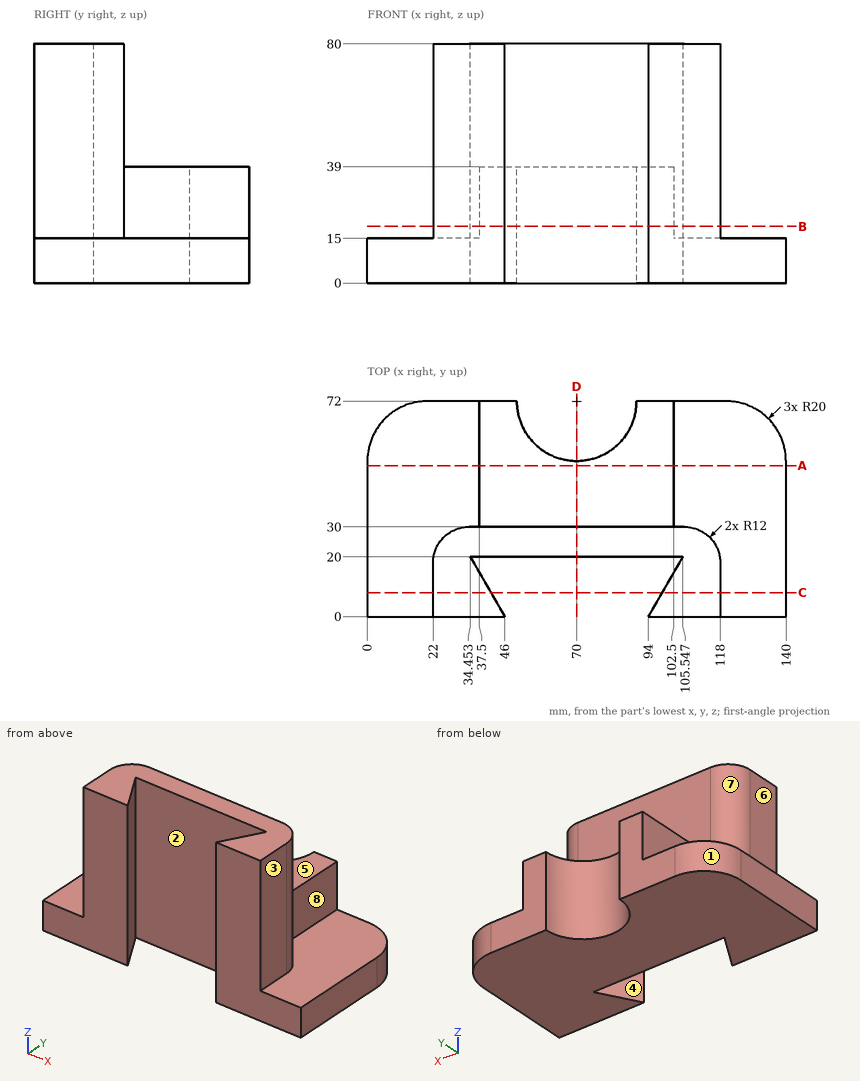
Could you check a few things on this drawing? It's one solid part, dimensions in mm from its lowest x, y, z. A direction names the side the tool comes from. Round coordinates to 2 decimals unless told otherwise and drop trailing zeros. Order: outer loops, then holes, each group sorted by start corner. A loop starts at its lowest first (then second) coordinate and runs counter-clockwise, first axis right, second up. Notation, with made-up numbers: M 42.5,37 L 76.5,37 A29 cw 76.5,76 Z; hole C 61,-5 d2. An arc over 180 degrees is marked long. Return JSON: item names as keys, results as strings. Group by question number.
1. I'm going to push flat-ended pins straight in: pin 1 Ø7 at (y, z) = (56.5, 29.5) entering from +X; pin 2 Ø12 at (x, y) = (59.5, 38) entering from -Z; pin 3 Ø12 at (y, z) = (48, 27) entering from -X; pin 4 Ø5.5 at (y, z) = (5.5, 42.5) entering from +X. Where does each tip first touch, or does it pass through?
2. If we section it at A-A on y = 50.5: List the corners of the cut face in (x, z) for me, then the cut area to 3 significant figures.
3. If we section it at B-B on z = 19: List the corners of the cut face in (x, y) for me.
4. If we mould it in two halves opening along Y, with no side actions, what happens to the marked faces 1, 2 and 3? For each: pulls with the +Y half, pulls with the -Y half, needs draft (parallel to the pull), parting line crosses it, or undercut.
5. Please list where these lines run through material, in increasing order: probe 1 along Y at (x, z) = (84.5, 62); probe 2 along X at (y, z) = (14.5, 11); probe 3 along Z at (x, y) = (72, 36).
6. On a 3-axis mill with a long thin cutter (end or side, diameter ignored), from which of +Z, -Z, +X, -X, +Y, -Y can I reach the whole of each face in a straight line? I mean the marked faces 4, 5, 6, 7 and 8. Say none if no direction works.
7. If we section it at C-C on y = 8: List the corners of the cut face in (x, z) for me.
8. If we section it at D-D on x = 70: List the corners of the cut face in (y, z) for me, then the cut area to 3 significant figures.
Reply:
{
 "1": {"pin 1": "x = 102.5", "pin 2": "z = 0", "pin 3": "x = 37.5", "pin 4": "x = 118"},
 "2": {"outline": "M 0,0 L 140,0 L 140,15 L 102.5,15 L 102.5,39 L 37.5,39 L 37.5,15 L 0,15 Z", "area": "3,660 mm^2"},
 "3": {"outline": "M 22,0 L 46,0 L 34.45,20 L 105.55,20 L 94,0 L 118,0 L 118,18 A12 ccw 106,30 L 102.5,30 L 102.5,72 L 90,72 A20 cw 50,72 L 37.5,72 L 37.5,30 L 34,30 A12 ccw 22,18 Z"},
 "4": {"face 1": "pulls with the +Y half", "face 2": "undercut", "face 3": "needs draft"},
 "5": {"probe 1": "20 to 30", "probe 2": "0 to 37.63, 102.37 to 140", "probe 3": "0 to 39"},
 "6": {"face 4": "+Z, -Z", "face 5": "+Z, +X, -X, +Y", "face 6": "+Z, -X, +Y, -Y", "face 7": "+Z, -X, +Y", "face 8": "+Z, +X, +Y"},
 "7": {"outline": "M 0,0 L 41.38,0 L 41.38,80 L 22,80 L 22,15 L 0,15 Z; M 98.62,0 L 140,0 L 140,15 L 118,15 L 118,80 L 98.62,80 Z"},
 "8": {"outline": "M 20,0 L 52,0 L 52,39 L 30,39 L 30,80 L 20,80 Z", "area": "1,660 mm^2"}
}
